```python
from build123d import *

# Parameters (mm, degrees)
SKETCH1_R               = 50
SKETCH1_R_2             = 37.5
BOSS_EXTRUDE1_DEPTH     = 25
BOSS_EXTRUDE2_DEPTH     = 87.5
CUT_EXTRUDE1_DEPTH      = 201.390244274
CUT_EXTRUDE1_DEPTH_BACK = 201.390244274
SKETCH3_W               = 75
SKETCH3_H               = 130
SKETCH4_R               = 15
CUT_EXTRUDE2_DEPTH      = 165.487841496
SKETCH5_R               = 20
CUT_EXTRUDE3_DEPTH      = 236.849528301


with BuildPart() as part:
    # Sketch1 → Boss-Extrude1 (new body)
    with BuildSketch(Plane(origin=(0, 0, 0), x_dir=(1, 0, 0), z_dir=(0, 1, 0))):
        with Locations(Location((0, 0, 0), (0, 0, 270))):
            Circle(SKETCH1_R)
        with Locations(Location((0, 0, 0), (0, 0, 270))):
            Circle(SKETCH1_R_2, mode=Mode.SUBTRACT)
    extrude(amount=-BOSS_EXTRUDE1_DEPTH)

    # Sketch2 → Boss-Extrude2 (add, symmetric)
    with BuildSketch(Plane(origin=(0, 0, 0), x_dir=(0, 0, -1), z_dir=(1, 0, 0))):
        with BuildLine():
            Line((-50, 0), (50, 0))
            Line((50, 0), (50, 100))
            ThreePointArc((50, 100), (0, 150), (-50, 100))
            Line((-50, 100), (-50, 0))
        make_face()
    extrude(amount=BOSS_EXTRUDE2_DEPTH, both=True)

    # Sketch3 → Cut-Extrude1 (cut, two sides: drawn at the far end of the back side and taken through both)
    with BuildSketch(Plane.XY.offset(50).offset(-CUT_EXTRUDE1_DEPTH_BACK)):
        with Locations((0, 85)):
            Rectangle(SKETCH3_W, SKETCH3_H)
    extrude(amount=CUT_EXTRUDE1_DEPTH + CUT_EXTRUDE1_DEPTH_BACK, mode=Mode.SUBTRACT)

    # Sketch4 → Cut-Extrude2 (cut, through all)
    with BuildSketch(Plane(origin=(0, 20, 0), x_dir=(1, 0, 0), z_dir=(0, 1, 0))):
        with Locations(Location((0, 0, 0), (0, 0, 180))):
            Circle(SKETCH4_R)
    extrude(amount=-CUT_EXTRUDE2_DEPTH, mode=Mode.SUBTRACT)

    # Sketch5 → Cut-Extrude3 (cut, through all)
    with BuildSketch(Plane(origin=(87.5, 0, 0), x_dir=(0, 0, -1), z_dir=(1, 0, 0))):
        with Locations((0, 100)):
            Circle(SKETCH5_R)
    extrude(amount=-CUT_EXTRUDE3_DEPTH, mode=Mode.SUBTRACT)


solid = part.part
```
Could you check a few things on this model? Use its own coordinates, in mm. A direction names the side the tool comes from. Round coordinates to 2 decimals unless told otherwise and drop trailing zeros. Write each loop counter-clockwise with the first axis right and the second up, starting at its lowest first coordinate (ties: lowest second). Pieces come first, ordered by that corner, then holes. Notation, with made-up numbers: M -32.75,49 L -15.75,49 A7 ccw -15.75,58 Z; hole C -15.5,38 d3. An arc over 180 degrees is marked long. Write each question's results on one line, items separated by ' | '. Start each with the question number.
1. On a 3-axis mill with a long thin cutter (end or side, diameter ignored), from which of +Z, -Z, +X, -X, +Y, -Y can I reach the whole of each face in a straight line? I mean faces 1 (the face through (16, 20, -1)), 2 (the face through (37, -25, 7)), 3 (the face through (15.02, -12.32, 47.69)). Say none if no direction works.
2. I'm going to push flat-ended pins straight in: pin 1 Ø3 at (x, z) = (33.5, 8.5) entering from +Y; pin 2 Ø2 at (x, y) = (44, 120) entering from +Z; pin 3 Ø10 at (x, z) = (-59.5, 34.5) entering from +Y. Where does each tip first touch, or does it pass through?
3. I need wall thicknesses on L1, parallel to Z at x = 80, y = 100.5; L2, parallel to Y at x = -76, z = 0; L3, parallel to X at y = 127.5, z = -30.5. Which ranges of each line are inside material? Lowest first, please. Write a range as from..to.
4. Thinking about a two-plate mould opening in X: for faces 4 (the face through (87.5, 76, 1)), 5 (the face through (-37.5, 70, -1)), 6 (the face through (-62.15, 149.988, -1.099)), 7 (the face through (-16, 0, 1)), which applies, +X half, -X half, draft (parallel to the pull), parting line (faces both ways), or undercut?
5. Imagine slicing it at D-D on z = -28. List the corners of the cut face in (x, y) for me.
6. Imagine slicing it at C-C on x = 69.5. List the corners of the cut face in (y, z) for me, and give its area (3 significant figures).
7. Imagine slicing it at B-B on z = 0. List the corners of the cut face in (x, y) for me, and give its area (3 significant figures).
8. Imagine slicing it at A-A on y = 75. List the corners of the cut face in (x, z) for me.
Result sheet:
1) face 1: +Z, -Z, +Y | face 2: +Z, -Z, +X, -X, -Y | face 3: -Y
2) pin 1: stops at y = 20 | pin 2: stops at z = 46.25 | pin 3: stops at y = 140.37
3) L1: z = -50..-19.99, 19.99..50 | L2: y = 0..80, 120..150 | L3: x = -87.5..-37.5, 37.5..87.5
4) face 4: +X half | face 5: undercut | face 6: draft | face 7: undercut
5) outline: M -87.5,0 L -41.42,0 L -41.42,-25 L -24.94,-25 L -24.94,0 L 24.94,0 L 24.94,-25 L 41.42,-25 L 41.42,0 L 87.5,0 L 87.5,141.42 L 37.5,141.42 L 37.5,20 L -37.5,20 L -37.5,141.42 L -87.5,141.42 Z
6) outline: M 0,-50 L 100,-50 A50 ccw 100,50 L 0,50 Z; hole C 100,0 d40 | area: 12,700 mm^2
7) outline: M -87.5,0 L -50,0 L -50,-25 L -37.5,-25 L -37.5,0 L -15,0 L -15,20 L -37.5,20 L -37.5,80 L -87.5,80 Z; M -87.5,120 L -37.5,120 L -37.5,150 L -87.5,150 Z; M 15,0 L 37.5,0 L 37.5,-25 L 50,-25 L 50,0 L 87.5,0 L 87.5,80 L 37.5,80 L 37.5,20 L 15,20 Z; M 37.5,120 L 87.5,120 L 87.5,150 L 37.5,150 Z | area: 12,500 mm^2
8) outline: M -87.5,-50 L -37.5,-50 L -37.5,50 L -87.5,50 Z; M 37.5,-50 L 87.5,-50 L 87.5,50 L 37.5,50 Z
